Read the model definition and answer for the solid it produces. Units are mm, in the model's axes. Coordinates: 2 decimals unless noted, no trailing zeros. Order: outer loops, then holes, each group sorted by start corner. A loop starts at its lowest first (then second) coordinate and runs counter-clockwise, first axis right, second up.
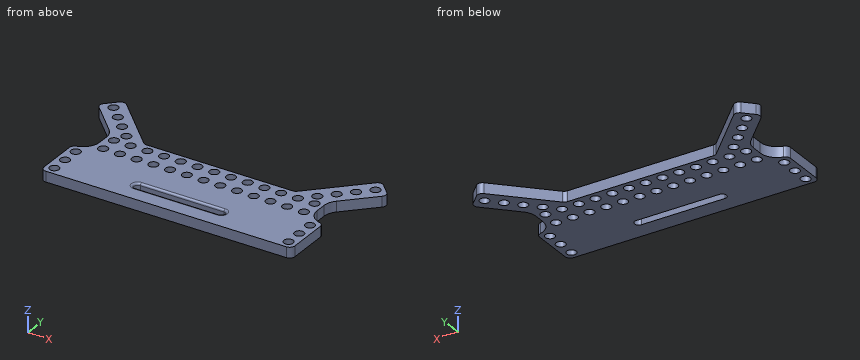
from build123d import *

# Parameters (mm, degrees)
SKETCH_1_R      = 2.25
EXTRUDE_1_DEPTH = 5
FILLET_1_R      = 2.5
FILLET_2_R      = 1
FILLET_3_R      = 8


with BuildPart() as part:
    # 草图1 → 凸台-拉伸1 (new body)
    with BuildSketch(Plane.XY):
        Polygon((-60, 4), (-60, -20), (60, -20), (60, 4), (52, 4), (52, 20), (69.455844123, 37.455844123), (61.455844123, 45.455844123), (36, 20), (-36, 20), (-61.455844123, 45.455844123), (-69.455844123, 37.455844123), (-52, 20), (-52, 4), align=None)
        with Locations((-56, -16)):
            Circle(SKETCH_1_R, mode=Mode.SUBTRACT)
        with Locations((-56, -8)):
            Circle(SKETCH_1_R, mode=Mode.SUBTRACT)
        with Locations((-56, 0)):
            Circle(SKETCH_1_R, mode=Mode.SUBTRACT)
        with Locations((56, 0)):
            Circle(SKETCH_1_R, mode=Mode.SUBTRACT)
        with Locations((56, -16)):
            Circle(SKETCH_1_R, mode=Mode.SUBTRACT)
        with Locations((56, -8)):
            Circle(SKETCH_1_R, mode=Mode.SUBTRACT)
        with Locations((-48, 16)):
            Circle(SKETCH_1_R, mode=Mode.SUBTRACT)
        with Locations((-48, 8)):
            Circle(SKETCH_1_R, mode=Mode.SUBTRACT)
        with Locations((-40, 16)):
            Circle(SKETCH_1_R, mode=Mode.SUBTRACT)
        with Locations((-40, 8)):
            Circle(SKETCH_1_R, mode=Mode.SUBTRACT)
        with Locations((-32, 16)):
            Circle(SKETCH_1_R, mode=Mode.SUBTRACT)
        with Locations((-32, 8)):
            Circle(SKETCH_1_R, mode=Mode.SUBTRACT)
        with Locations((-24, 16)):
            Circle(SKETCH_1_R, mode=Mode.SUBTRACT)
        with Locations((-24, 8)):
            Circle(SKETCH_1_R, mode=Mode.SUBTRACT)
        with Locations((-16, 16)):
            Circle(SKETCH_1_R, mode=Mode.SUBTRACT)
        with Locations((-16, 8)):
            Circle(SKETCH_1_R, mode=Mode.SUBTRACT)
        with Locations((-8, 16)):
            Circle(SKETCH_1_R, mode=Mode.SUBTRACT)
        with Locations((-8, 8)):
            Circle(SKETCH_1_R, mode=Mode.SUBTRACT)
        with Locations((0, 16)):
            Circle(SKETCH_1_R, mode=Mode.SUBTRACT)
        with Locations((0, 8)):
            Circle(SKETCH_1_R, mode=Mode.SUBTRACT)
        with Locations((8, 16)):
            Circle(SKETCH_1_R, mode=Mode.SUBTRACT)
        with Locations((8, 8)):
            Circle(SKETCH_1_R, mode=Mode.SUBTRACT)
        with Locations((16, 16)):
            Circle(SKETCH_1_R, mode=Mode.SUBTRACT)
        with Locations((16, 8)):
            Circle(SKETCH_1_R, mode=Mode.SUBTRACT)
        with Locations((24, 16)):
            Circle(SKETCH_1_R, mode=Mode.SUBTRACT)
        with Locations((24, 8)):
            Circle(SKETCH_1_R, mode=Mode.SUBTRACT)
        with Locations((32, 16)):
            Circle(SKETCH_1_R, mode=Mode.SUBTRACT)
        with Locations((32, 8)):
            Circle(SKETCH_1_R, mode=Mode.SUBTRACT)
        with Locations((40, 16)):
            Circle(SKETCH_1_R, mode=Mode.SUBTRACT)
        with Locations((40, 8)):
            Circle(SKETCH_1_R, mode=Mode.SUBTRACT)
        with Locations((48, 16)):
            Circle(SKETCH_1_R, mode=Mode.SUBTRACT)
        with Locations((48, 8)):
            Circle(SKETCH_1_R, mode=Mode.SUBTRACT)
        with Locations((-45.656854249, 21.656854249)):
            Circle(SKETCH_1_R, mode=Mode.SUBTRACT)
        with Locations((-51.313708499, 27.313708499)):
            Circle(SKETCH_1_R, mode=Mode.SUBTRACT)
        with Locations((-56.970562748, 32.970562748)):
            Circle(SKETCH_1_R, mode=Mode.SUBTRACT)
        with Locations((-62.627416998, 38.627416998)):
            Circle(SKETCH_1_R, mode=Mode.SUBTRACT)
        with Locations((45.656854249, 21.656854249)):
            Circle(SKETCH_1_R, mode=Mode.SUBTRACT)
        with Locations((51.313708499, 27.313708499)):
            Circle(SKETCH_1_R, mode=Mode.SUBTRACT)
        with Locations((56.970562748, 32.970562748)):
            Circle(SKETCH_1_R, mode=Mode.SUBTRACT)
        with Locations((62.627416998, 38.627416998)):
            Circle(SKETCH_1_R, mode=Mode.SUBTRACT)
        with BuildLine():
            Line((20, -8), (-20, -8))
            ThreePointArc((-20, -8), (-22, -10), (-20, -12))
            Line((-20, -12), (20, -12))
            ThreePointArc((20, -12), (22, -10), (20, -8))
        make_face(mode=Mode.SUBTRACT)
    extrude(amount=EXTRUDE_1_DEPTH)

    # 圆角1
    fillet_1_edges = [part.edges().sort_by_distance(p)[0] for p in [
        (60, 4, 2.5),
        (60, -20, 2.5),
        (-60, -20, 2.5),
        (-60, 4, 2.5),
        (-69.455844123, 37.455844123, 2.5),
        (-61.455844123, 45.455844123, 2.5),
        (-36, 20, 2.5),
        (36, 20, 2.5),
        (61.455844123, 45.455844123, 2.5),
        (69.455844123, 37.455844123, 2.5),
    ]]
    fillet(fillet_1_edges, radius=FILLET_1_R)

    # 圆角2
    fillet_2_edges = [part.edges().sort_by_distance(p)[0] for p in [
        (0, -8, 5),
        (22, -10, 5),
        (0, -12, 5),
        (-22, -10, 5),
    ]]
    fillet(fillet_2_edges, radius=FILLET_2_R)

    # 圆角3
    fillet_3_edges = [part.edges().sort_by_distance(p)[0] for p in [
        (-52, 4, 2.5),
        (-52, 20, 2.5),
        (52, 4, 2.5),
        (52, 20, 2.5),
    ]]
    fillet(fillet_3_edges, radius=FILLET_3_R)


solid = part.part
Q1. The part is cut by section A-A, the plane y = -16. Determine the outline of the cut face in (x, z), then the cut area to 3 significant figures.
Q2. Straight lines are drawn through the part: L1, parallel to Y at x = 0, z = 2.3; L2, parallel to X at y = 28, z = 1.3; L3, parallel to Y at x = 59, z = 2.65. For each, find the intervals that lie inside material, in ascending order.
Q3. The part is cut by section C-C, the plane x = 31. Determine the outline of the cut face in (y, z), then the cut area to 3 significant figures.
Q4. The part is cut by section B-B, the plane x = 8. Determine the outline of the cut face in (y, z), then the cut area to 3 significant figures.
Q5. The part is cut by section D-D, the plane z = 2.85. State how many separate pieces and enclosed holes the cut face has, then the cut area to 3 significant figures.
Q6. Each of these flat-tipped pins is pushed along its axis until it touches: P1, Ø5, axis at x = -62.63, y = 38.63, coming from the -Z side; P2, Ø3.5, axis at x = 16, y = 8, coming from the -Z side; P3, Ø1, axis at y = 1.5, z = 1, coming from the +X side; P4, Ø3, axis at x = -51.5, z = 3.5, coming from the +Y side. Where does it stop, or does it pass through?
Computed values:
1. outline: (-60, 0) - (-58.25, 0) - (-58.25, 5) - (-60, 5) - close; (-53.75, 0) - (53.75, 0) - (53.75, 5) - (-53.75, 5) - close; (58.25, 0) - (60, 0) - (60, 5) - (58.25, 5) - close
1. area: 555 mm2
2. L1: y = -20 to -12, -8 to 5.75, 10.25 to 13.75, 18.25 to 20
2. L2: x = -60 to -53.46, -49.17 to -44, 44 to 49.17, 53.46 to 60
2. L3: y = -19.5 to 3.5, 27 to 32, 33.94 to 43
3. outline: (-20, 0) - (5.98, 0) - (5.98, 5) - (-20, 5) - close; (10.02, 0) - (13.98, 0) - (13.98, 5) - (10.02, 5) - close; (18.02, 0) - (20, 0) - (20, 5) - (18.02, 5) - close
3. area: 160 mm2
4. outline: (-20, 0) - (-12, 0) - (-12, 4) arc R1 ccw to (-13, 5) - (-20, 5) - close; (-8, 0) - (5.75, 0) - (5.75, 5) - (-7, 5) arc R1 ccw to (-8, 4) - close; (10.25, 0) - (13.75, 0) - (13.75, 5) - (10.25, 5) - close; (18.25, 0) - (20, 0) - (20, 5) - (18.25, 5) - close
4. area: 135 mm2
5. separate pieces: 1
5. enclosed holes: 41
5. area: 4,440 mm2
6. P1: stops at z = 0
6. P2: passes through
6. P3: stops at x = 60
6. P4: stops at y = 37
